```python
from build123d import *

# Parameters (mm, degrees)
BOSS_EXTRUDE1_DEPTH                 = 30
BOSS_EXTRUDE2_DEPTH                 = 25
CUT_EXTRUDE9_DEPTH                  = 28.6
BOSS_EXTRUDE10_DEPTH                = 4
F_3_5_3_5_DIAMETER_HOLE1_AT_2_COUNT = 2
F_3_5_3_5_DIAMETER_HOLE1_AT_2_PITCH = 14.509439018
F_3_5_3_5_DIAMETER_HOLE2_AT_2_COUNT = 2
F_3_5_3_5_DIAMETER_HOLE2_AT_2_PITCH = 16
F_4_0MM_DOWEL_HOLE1_D               = 3.5
BOSS_EXTRUDE11_DEPTH                = 6.4
F_4_0MM_DOWEL_HOLE2_D               = 3.5
F_4_0MM_DOWEL_HOLE2_DEPTH           = 5
F_3_0MM_DOWEL_HOLE1_D               = 3.5
BOSS_EXTRUDE13_DEPTH                = 5
F_3_0MM_DOWEL_HOLE2_D               = 3.5
F_3_0MM_DOWEL_HOLE2_DEPTH           = 5
BOSS_EXTRUDE14_START                = 28
BOSS_EXTRUDE14_DEPTH                = 22.6
BOSS_EXTRUDE14_2_DEPTH              = 2
BOSS_EXTRUDE14_START_2              = 48.6
BOSS_EXTRUDE14_3_DEPTH              = 2
BOSS_EXTRUDE15_START                = 28
BOSS_EXTRUDE15_DEPTH                = 22.6
BOSS_EXTRUDE15_2_DEPTH              = 2
BOSS_EXTRUDE15_START_2              = 48.6
BOSS_EXTRUDE15_3_DEPTH              = 2
SKETCH54_W                          = 6
SKETCH54_H                          = 11
BOSS_EXTRUDE16_DEPTH                = 3
CUT_EXTRUDE10_DEPTH                 = 3


# Read off the part's stored shape, not the designer's step: Boss-Extrude14, Boss-Extrude15
with BuildPart() as part:
    # Sketch1 → Boss-Extrude1 (new body)
    with BuildSketch(Plane.XY):
        Polygon((-83.548089297, 0), (83.548089297, 0), (83.548089297, -11), (97.64, -11), (96.548089297, -8), (86.548089297, -8), (86.548089297, 19.474774195), (77.1187914, 45.381557247), (74.299713538, 44.355496817), (83.548089297, 18.945793252), (83.548089297, 5), (-83.548089297, 5), (-83.548089297, 18.945793252), (-74.299713538, 44.355496817), (-77.1187914, 45.381557247), (-86.548089297, 19.474774195), (-86.548089297, -8), (-96.548089297, -8), (-97.64, -11), (-83.548089297, -11), align=None)
    extrude(amount=BOSS_EXTRUDE1_DEPTH)

    # Sketch2 → Boss-Extrude2 (add)
    with BuildSketch(Plane.XY.offset(30)):
        Polygon((-77.1187914, 45.381557247), (-74.299713538, 44.355496817), (-83.548089297, 18.945793252), (-83.548089297, 5), (-63.548089297, 5), (-63.548089297, 0), (-86.548089297, 0), (-86.548089297, 19.474774195), align=None)
        Polygon((77.1187914, 45.381557247), (74.299713538, 44.355496817), (83.548089297, 18.945793252), (83.548089297, 5), (63.548089297, 5), (63.548089297, 0), (86.548089297, 0), (86.548089297, 19.474774195), align=None)
    extrude(amount=BOSS_EXTRUDE2_DEPTH)

    # Sketch26 → Cut-Extrude9 (cut)
    with BuildSketch(Plane.ZY.offset(86.548089297)):
        Polygon((0, 45.381557247), (32.311383976, 45.381557247), (0, 6.874349312), align=None)
    cut_extrude9 = extrude(amount=-CUT_EXTRUDE9_DEPTH, mode=Mode.SUBTRACT)

    # Mirror1: Cut-Extrude9 across plane
    add(cut_extrude9.mirror(Plane.ZY), mode=Mode.SUBTRACT)

    # Sketch27 → Boss-Extrude10 (add)
    with BuildSketch(Plane(origin=(0, 2.840315541, -3.38495625), x_dir=(-1, 0, 0), z_dir=(0, 0.6427876096865439, -0.7660444431189742))):
        Polygon((-86.548089297, 21.024208003), (-52.1187914, 21.024208003), (-52.1187914, 55.533647021), (-77.1187914, 55.533647021), align=None)
    boss_extrude10 = extrude(amount=-BOSS_EXTRUDE10_DEPTH)

    # Sketch32 → Ø3.5 (3.5) Diameter Hole1 (revolve, cut)
    with BuildSketch(Plane(origin=(62.1187914, 37.721112816, 25.883507879), x_dir=(0, 0.7660444431189745, 0.6427876096865438), z_dir=(1, 0, 0))):
        Polygon((0, 0), (0, 6.051506083), (1.75, 5), (1.75, 0), align=None)
    f_3_5_3_5_diameter_hole1 = revolve(axis=Axis((62.1187914, 41.802814137, 21.019125665), (0, -0.6427876096865437, 0.7660444431189743)), mode=Mode.SUBTRACT)

    # Ø3.5 (3.5) Diameter Hole1 at 2: Ø3.5 (3.5) Diameter Hole1 ×2
    with Locations(*[Vector(0, -0.7660444431189745, -0.6427876096865437) * (i * F_3_5_3_5_DIAMETER_HOLE1_AT_2_PITCH) for i in range(1, F_3_5_3_5_DIAMETER_HOLE1_AT_2_COUNT)]):
        add(f_3_5_3_5_diameter_hole1, mode=Mode.SUBTRACT)

    # Mirror12: Boss-Extrude10, Ø3.5 (3.5) Diameter Hole1 across plane
    add(boss_extrude10.mirror(Plane.ZY))
    add(f_3_5_3_5_diameter_hole1.mirror(Plane.ZY), mode=Mode.SUBTRACT)

    # Mirror12 copy 1 sketch → Mirror12 copy 1 (revolve, cut)
    with BuildSketch(Plane(origin=(-62.1187914, 26.606237684, 16.557020255), x_dir=(0, 0.7660444431189745, 0.6427876096865438), z_dir=(-1, 0, 0))):
        Polygon((0, 0), (0, -6.051506083), (1.75, -5), (1.75, 0), align=None)
    revolve(axis=Axis((-62.1187914, 30.687939005, 11.692638041), (0, 0.6427876096865437, -0.7660444431189743)), mode=Mode.SUBTRACT)

    # Sketch36 → Ø3.5 (3.5) Diameter Hole2 (revolve, cut)
    with BuildSketch(Plane(origin=(91.548089297, -8, 7), x_dir=(0, 0, 1), z_dir=(1, 0, 0))):
        Polygon((0, 0), (0, 6.051506083), (1.75, 5), (1.75, 0), align=None)
    f_3_5_3_5_diameter_hole2 = revolve(axis=Axis((91.548089297, -1.65, 7), (0, -1, 0)), mode=Mode.SUBTRACT)

    # Ø3.5 (3.5) Diameter Hole2 at 2: Ø3.5 (3.5) Diameter Hole2 ×2
    with Locations(*[(0, 0, i * F_3_5_3_5_DIAMETER_HOLE2_AT_2_PITCH) for i in range(1, F_3_5_3_5_DIAMETER_HOLE2_AT_2_COUNT)]):
        add(f_3_5_3_5_diameter_hole2, mode=Mode.SUBTRACT)

    # Mirror13: Ø3.5 (3.5) Diameter Hole2 across plane
    add(f_3_5_3_5_diameter_hole2.mirror(Plane.ZY), mode=Mode.SUBTRACT)

    # Mirror13 copy 1 sketch → Mirror13 copy 1 (revolve, cut)
    with BuildSketch(Plane(origin=(-91.548089297, -8, 23), x_dir=(0, 0, 1), z_dir=(-1, 0, 0))):
        Polygon((0, 0), (0, -6.051506083), (1.75, -5), (1.75, 0), align=None)
    revolve(axis=Axis((-91.548089297, -1.65, 23), (0, 1, 0)), mode=Mode.SUBTRACT)

    # Sketch37 → Ø3.5 (3.5) Diameter Hole3 (revolve, cut)
    with BuildSketch(Plane(origin=(80.538992834, 35.984631039, 45), x_dir=(-0.342020143325673, 0.9396926207859069, 0), z_dir=(0, 0, 1))):
        Polygon((0, 0), (0, 6.051506083), (1.75, 5), (1.75, 0), align=None)
    f_3_5_3_5_diameter_hole3 = revolve(axis=Axis((86.506040976, 38.156458949, 45), (-0.9396926207859069, -0.34202014332567293, 0)), mode=Mode.SUBTRACT)

    # Mirror14: Ø3.5 (3.5) Diameter Hole3 across plane
    add(f_3_5_3_5_diameter_hole3.mirror(Plane.ZY), mode=Mode.SUBTRACT)

    # Ø4.0mm Dowel Hole1 (through all)
    with Locations(Plane(origin=(0, 5, 0), x_dir=(1, 0, 0), z_dir=(0, 1, 0))):
        with Locations((-12.7, -4), (12.7, -4)):
            Hole(F_4_0MM_DOWEL_HOLE1_D / 2)

    # Sketch44 → Boss-Extrude11 (add)
    with BuildSketch(Plane.XY.offset(55)):
        Polygon((86.548089297, 0), (86.548089297, -8), (96.548089297, -8), (97.64, -11), (86.548089297, -11), (83.548089297, -11), (83.548089297, 5), (86.548089297, 5), align=None)
    boss_extrude11 = extrude(amount=-BOSS_EXTRUDE11_DEPTH)

    # Mirror15: Boss-Extrude11 across plane
    add(boss_extrude11.mirror(Plane.ZY))

    # Ø4.0mm Dowel Hole2
    with Locations(Plane(origin=(0, 5, 0), x_dir=(1, 0, 0), z_dir=(0, 1, 0))):
        with Locations((79.548089297, -52), (79.548089297, -26.6)):
            f_4_0mm_dowel_hole2 = Hole(F_4_0MM_DOWEL_HOLE2_D / 2, depth=F_4_0MM_DOWEL_HOLE2_DEPTH)

    # Ø3.0mm Dowel Hole1 (through all)
    with Locations(Plane(origin=(0, 5, 0), x_dir=(1, 0, 0), z_dir=(0, 1, 0))):
        with Locations((47.7, -4), (25.702954744, -16.7)):
            f_3_0mm_dowel_hole1 = Hole(F_3_0MM_DOWEL_HOLE1_D / 2)

    # Mirror17: Ø4.0mm Dowel Hole2, Ø3.0mm Dowel Hole1 across plane
    add(f_4_0mm_dowel_hole2.mirror(Plane.ZY), mode=Mode.SUBTRACT)
    add(f_3_0mm_dowel_hole1.mirror(Plane.ZY), mode=Mode.SUBTRACT)

    # Sketch49 → Boss-Extrude13 (add)
    with BuildSketch(Plane(origin=(0, 5, 0), x_dir=(1, 0, 0), z_dir=(0, 1, 0))):
        Polygon((-41.897454203, -30), (-63.548089297, -42.5), (-63.548089297, -30), align=None)
    boss_extrude13 = extrude(amount=-BOSS_EXTRUDE13_DEPTH)

    # Mirror18: Boss-Extrude13 across plane
    add(boss_extrude13.mirror(Plane.ZY))

    # Ø3.0mm Dowel Hole2
    with Locations(Plane(origin=(0, 5, 0), x_dir=(1, 0, 0), z_dir=(0, 1, 0))):
        with Locations((-63.548089297, -10), (-50.848089297, -31.997045256)):
            f_3_0mm_dowel_hole2 = Hole(F_3_0MM_DOWEL_HOLE2_D / 2, depth=F_3_0MM_DOWEL_HOLE2_DEPTH)

    # Mirror19: Ø3.0mm Dowel Hole2 across plane
    add(f_3_0mm_dowel_hole2.mirror(Plane.ZY), mode=Mode.SUBTRACT)

    # Boss-Extrude14 outline → Boss-Extrude14 (add)
    with BuildSketch(Plane.XY.offset(BOSS_EXTRUDE14_START)):
        Polygon((93.636327423, 0), (92.908386955, 2), (86.548089297, 2), (86.548089297, 0), align=None)
    extrude(amount=BOSS_EXTRUDE14_DEPTH)

    # Boss-Extrude14 2 outline → Boss-Extrude14 2 (add)
    with BuildSketch(Plane.XY.offset(BOSS_EXTRUDE14_START)):
        Polygon((96.548089297, -8), (93.636327423, 0), (86.548089297, 0), (86.548089297, -8), align=None)
    extrude(amount=BOSS_EXTRUDE14_2_DEPTH)

    # Boss-Extrude14 3 outline → Boss-Extrude14 3 (add)
    with BuildSketch(Plane.XY.offset(BOSS_EXTRUDE14_START_2)):
        Polygon((96.548089297, -8), (93.636327423, 0), (86.548089297, 0), (86.548089297, -8), align=None)
    extrude(amount=BOSS_EXTRUDE14_3_DEPTH)

    # Boss-Extrude15 outline → Boss-Extrude15 (add)
    with BuildSketch(Plane.XY.offset(BOSS_EXTRUDE15_START)):
        Polygon((-86.548089297, 2), (-92.903986965, 2), (-93.631927434, 0), (-86.548089297, 0), align=None)
    extrude(amount=BOSS_EXTRUDE15_DEPTH)

    # Boss-Extrude15 2 outline → Boss-Extrude15 2 (add)
    with BuildSketch(Plane.XY.offset(BOSS_EXTRUDE15_START)):
        Polygon((-86.548089297, 0), (-93.631927434, 0), (-96.543689308, -8), (-86.548089297, -8), align=None)
    extrude(amount=BOSS_EXTRUDE15_2_DEPTH)

    # Boss-Extrude15 3 outline → Boss-Extrude15 3 (add)
    with BuildSketch(Plane.XY.offset(BOSS_EXTRUDE15_START_2)):
        Polygon((-86.548089297, 0), (-93.631927434, 0), (-96.543689308, -8), (-86.548089297, -8), align=None)
    extrude(amount=BOSS_EXTRUDE15_3_DEPTH)

    # Sketch54 → Boss-Extrude16 (add)
    with BuildSketch(Plane(origin=(0, 0, 0), x_dir=(-1, 0, 0), z_dir=(0, 0, -1))):
        with Locations((-63.915800061, -5.5)):
            Rectangle(SKETCH54_W, SKETCH54_H)
    boss_extrude16 = extrude(amount=-BOSS_EXTRUDE16_DEPTH)

    # Sketch55 → Cut-Extrude10 (cut)
    with BuildSketch(Plane(origin=(0, 0, 0), x_dir=(-1, 0, 0), z_dir=(0, 0, -1))):
        with BuildLine():
            Line((-62.415800061, -3), (-62.415800061, -8))
            ThreePointArc((-62.415800061, -8), (-63.915800061, -9.5), (-65.415800061, -8))
            Line((-65.415800061, -8), (-65.415800061, -3))
            ThreePointArc((-65.415800061, -3), (-63.915800061, -1.5), (-62.415800061, -3))
        make_face()
    cut_extrude10 = extrude(amount=-CUT_EXTRUDE10_DEPTH, mode=Mode.SUBTRACT)

    # Mirror20: Boss-Extrude16, Cut-Extrude10 across plane
    add(boss_extrude16.mirror(Plane.ZY))
    add(cut_extrude10.mirror(Plane.ZY), mode=Mode.SUBTRACT)


solid = part.part
```
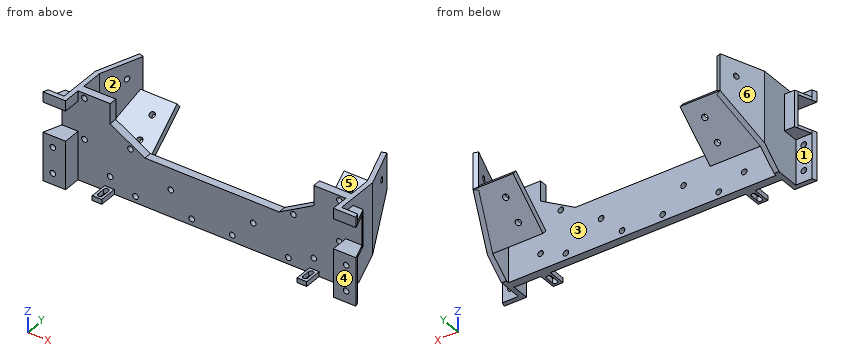
Input: part model. Units: mm. Frame: model coordinates. Face numbers are marked on the shaded views. A direction names the side the tool comes from. Give positions to 0.01 mm unless a question says otherwise; leave off trailing zeros. Order: outer loops, then holes, each group sorted by start corner. A loop starts at its lowest first (then second) coordinate and runs counter-clockwise, first axis right, second up.
1. Cut plane B-B (x = -57). Return loops of the section in (y, z).
Computed:
outline: (0, 0) - (5, 0) - (5, 38.72) - (0, 38.72) - close; (16.37, 13.19) - (18.95, 10.13) - (45.38, 32.31) - (42.81, 35.38) - close
2. Draft query along X for the marked faces 4, 5 and 6. Return one class per face: released by +X, released by -X, zero draft, split by the parting line, or undercut.
Computed:
face 4: zero draft
face 5: undercut
face 6: released by -X
3. Set-up query: the marked faces 1, 2 and 3. Return all of +Z, -Z, +X, -X, +Y, -Y with unobstructed straight access to the full face (end or side cutting, diameter ignored); none if empty.
Computed:
face 1: -Z, -X, +Y
face 2: +Z
face 3: +Z, -Z
4. Cut plane C-C (x = -21). Return loops of the section in (y, z), and give its area (3 significant figures).
Computed:
outline: (0, 0) - (5, 0) - (5, 30) - (0, 30) - close
area: 150 mm2
5. Cut plane A-A (z = 23). State how many separate pieces and enclosed holes the cut face has, and give its area (3 significant figures).
Computed:
separate pieces: 3
enclosed holes: 0
area: 1,490 mm2
6. Line query: probe 1 along X at (y, z) = (1, 10); probe 2 along Z at (x, y) = (87, -7); probe 3 along X at (y, z) = (19, 21). Output: solid intervals per line, ascending.
Computed:
probe 1: x = -86.55 to -65.3, -61.8 to 61.8, 65.3 to 86.55
probe 2: z = 28 to 30, 48.6 to 50.6
probe 3: x = -86.55 to -83.53, 83.53 to 86.55
7. Pin query (flat end, axial travel): pin 1 Ø3.5 at (x, y) = (88.5, -5) entering from -Z; pin 2 Ø4 at (y, z) = (9.5, 15.5) entering from +X; pin 3 Ø3 at (x, z) = (-10, 23.5) entering from +Y; pin 4 Ø1.5 at (x, z) = (56, 39.5) entering from +Y (3 decimals). Return the tip coordinate at first contact, or that it passes through.
Computed:
pin 1: stops at z = 28
pin 2: stops at x = 86.55
pin 3: stops at y = 5
pin 4: passes through
